from build123d import *

# Parameters (mm, degrees)
BOSS_EXTRUDE1_DEPTH                             = 5
CSK_FOR_M3_FLAT_HEAD_MACHINE_SCREW1_D           = 3.4
CSK_FOR_M3_FLAT_HEAD_MACHINE_SCREW1_DEPTH       = 10
CSK_FOR_M3_FLAT_HEAD_MACHINE_SCREW1_CSINK_D     = 4.2
CSK_FOR_M3_FLAT_HEAD_MACHINE_SCREW1_CSINK_ANGLE = 90
CSK_FOR_M3_FLAT_HEAD_MACHINE_SCREW1_TIP         = 1.021463052
CUT_EXTRUDE1_DEPTH                              = 2.762
SKETCH9_W                                       = 5
SKETCH9_H                                       = 5
CUT_EXTRUDE3_DEPTH                              = 1.5
SKETCH10_W                                      = 2
SKETCH10_H                                      = 2
CUT_EXTRUDE4_DEPTH                              = 3
CUT_EXTRUDE5_DEPTH                              = 3
CUT_EXTRUDE6_DEPTH                              = 3


with BuildPart() as part:
    # Sketch1 → Boss-Extrude1 (new body)
    with BuildSketch(Plane(origin=(0, 0, 0), x_dir=(0, 0, -1), z_dir=(1, 0, 0))):
        with BuildLine():
            Line((-36.25, 0.243748214), (36.25, 0.243748214))
            Line((36.25, 0.243748214), (36.25, 58.993748214))
            Line((36.25, 58.993748214), (39.75, 58.993748214))
            ThreePointArc((39.75, 58.993748214), (42.25, 61.493748214), (39.75, 63.993748214))
            Line((39.75, 63.993748214), (36.25, 63.993748214))
            Line((36.25, 63.993748214), (-10.25, 63.993748214))
            Line((-10.25, 63.993748214), (-36.25, 18.993748214))
            Line((-36.25, 18.993748214), (-36.25, 0.243748214))
        make_face()
        Polygon((31.25, 5.243748214), (-31.25, 5.243748214), (-31.25, 17.653143244), (-18.920674634, 38.992360224), (-7.364317129, 58.993748214), (31.25, 58.993748214), align=None, mode=Mode.SUBTRACT)
    extrude(amount=BOSS_EXTRUDE1_DEPTH)

    # CSK for M3 Flat Head Machine Screw1
    with Locations(Plane.ZY):
        with Locations((-39.75, 61.493748214)):
            CounterSinkHole(CSK_FOR_M3_FLAT_HEAD_MACHINE_SCREW1_D / 2, CSK_FOR_M3_FLAT_HEAD_MACHINE_SCREW1_CSINK_D / 2, depth=CSK_FOR_M3_FLAT_HEAD_MACHINE_SCREW1_DEPTH, counter_sink_angle=CSK_FOR_M3_FLAT_HEAD_MACHINE_SCREW1_CSINK_ANGLE)
            with Locations((0, 0, -(CSK_FOR_M3_FLAT_HEAD_MACHINE_SCREW1_DEPTH + CSK_FOR_M3_FLAT_HEAD_MACHINE_SCREW1_TIP / 2))):  # 118° drill point
                Cone(0, CSK_FOR_M3_FLAT_HEAD_MACHINE_SCREW1_D / 2, CSK_FOR_M3_FLAT_HEAD_MACHINE_SCREW1_TIP, mode=Mode.SUBTRACT)

    # Sketch6 → Cut-Extrude1 (cut)
    with BuildSketch(Plane(origin=(5, 0, 0), x_dir=(0, 0, -1), z_dir=(1, 0, 0))):
        Polygon((33.25, 60.993748214), (33.25, 3.243748214), (-33.25, 3.243748214), (-33.25, 18.189385232), (-8.518590277, 60.993748214), align=None)
    extrude(amount=-CUT_EXTRUDE1_DEPTH, mode=Mode.SUBTRACT)

    # Sketch9 → Cut-Extrude3 (cut)
    with BuildSketch(Plane.XY.offset(36.25)):
        with Locations((2.5, 2.743748214)):
            Rectangle(SKETCH9_W, SKETCH9_H)
    extrude(amount=-CUT_EXTRUDE3_DEPTH, mode=Mode.SUBTRACT)

    # Sketch10 → Cut-Extrude4 (cut)
    with BuildSketch(Plane(origin=(5, 0, 0), x_dir=(0, 0, -1), z_dir=(1, 0, 0))):
        with Locations((33.75, 61.993748214)):
            Rectangle(SKETCH10_W, SKETCH10_H)
    extrude(amount=-CUT_EXTRUDE4_DEPTH, mode=Mode.SUBTRACT)

    # Sketch13 → Cut-Extrude5 (cut)
    with BuildSketch(Plane(origin=(5, 0, 0), x_dir=(0, 0, -1), z_dir=(1, 0, 0))):
        Polygon((-8.75000025, 62.993748214), (-6.75, 62.993748214), (-6.750000265, 61.993748214), (-8.75000025, 61.993988423), align=None)
        Polygon((-11.135106519, 60.46294286), (-10.134551324, 62.194673006), (-9.26868625, 61.694395408), (-10.269241446, 59.962665262), align=None)
    extrude(amount=-CUT_EXTRUDE5_DEPTH, mode=Mode.SUBTRACT)

    # Sketch15 → Cut-Extrude6 (cut)
    with BuildSketch(Plane(origin=(5, 0, 0), x_dir=(0, 0, -1), z_dir=(1, 0, 0))):
        Polygon((-33.188472136, 22.293656216), (-33.938888532, 20.994858606), (-32.640090922, 20.244442209), (-31.889674526, 21.543239819), align=None)
    extrude(amount=-CUT_EXTRUDE6_DEPTH, mode=Mode.SUBTRACT)


solid = part.part
Could you check a few things on this model? Use its own coordinates, in mm. A direction names the side the tool comes from. Round coordinates to 2 decimals unless told otherwise and drop trailing zeros. Write each loop counter-clockwise with the first axis right and the second up, starting at its lowest first coordinate (ties: lowest second). Pieces come first, ordered by that corner, then holes. Notation, with made-up numbers: (-24.5, 58.25) - (14.5, 58.25) arc R34 ccw to (14.5, 91.25) - close; hole circle Ø3 at (86, 25.5). An arc over 180 degrees is marked (long way). Put each result on its own line as item: value. Start each with the question number.
(1) I want a section at C-C, the plane x = 4. Give the number of separate pieces and of enclosed holes in the cut face, plus the area to 3 significant figures.
(2) Will these pins go through, and if not, where does the flat tip stop? pin 1 (1 mm diameter, centred on y = 56, z = 15.5, fed in from +X); pin 2 (1.8 mm diameter, centred on x = 1.5, y = 25, fed in from +Z); pin 3 (2 mm diameter, centred on x = 4, y = 29, fed in from +Z); pin 4 (2 mm diameter, centred on x = 4, y = 62, fed in from +Z).
(3) For faces 1 (the flat face through (4, 62.994, -34)), 2 (the cylindrical face through (2.46, 61.44, -42.25)), 3 (the flat face through (2, 3, 34.75)), which set-ups out of +Z, -Z, +X, -X, +Y, -Y let a thin tool reach every point of the face, with its end or its side?
(4) I want a section at B-B, the plane y = 49. Please give me the cut outline in (x, z), plus the area to 3 significant figures.
(5) I need wall thicknesses on probe 1 along Y at (x, z) = (4.1, 7); probe 2 along Y at (x, z) = (2.55, -39.75); probe 3 along Y at (x, z) = (1.85, -17.5). Which ranges of each line are inside material? Lowest first, please.
(6) Thinking about a two-plate mould opening in Z: for faces 4 (the flat face through (2.465, 41.809, 23.068)), 5 (the flat face through (1, 11, 31.25)), 6 (the flat face through (5, 46, 18)), which applies, released by +Z, released by -Z, zero draft, split by the parting line, or undercut?
(7) I want a section at A-A, the plane z = -21.5. Please give me the cut outline in (x, y), plus the area to 3 significant figures.
Here are the results:
1. separate pieces: 1
1. enclosed holes: 5
1. area: 726 mm^2
2. pin 1: passes through
2. pin 2: stops at z = 33.3
2. pin 3: stops at z = 31.05
2. pin 4: stops at z = 11.98
3. face 1: +X
3. face 2: -Z, +X, -X
3. face 3: +Z, +X, -X, -Y
4. outline: (0, -36.25) - (5, -36.25) - (5, -33.25) - (2.24, -33.25) - (2.24, -31.25) - (0, -31.25) - close; (0, 13.14) - (2.24, 13.14) - (2.24, 15.45) - (5, 15.45) - (5, 18.91) - (0, 18.91) - close
4. area: 42.0 mm^2
5. probe 1: y = 0.24 to 3.24, 60.99 to 61.99, 62.99 to 63.99
5. probe 2: y = 58.99 to 59.79, 63.19 to 63.99
5. probe 3: y = 0.24 to 5.24, 58.99 to 63.99
6. face 4: released by +Z
6. face 5: undercut
6. face 6: zero draft
7. outline: (0, 0.24) - (5, 0.24) - (5, 3.24) - (2.24, 3.24) - (2.24, 5.24) - (0, 5.24) - close; (0, 58.99) - (2.24, 58.99) - (2.24, 60.99) - (5, 60.99) - (5, 63.99) - (0, 63.99) - close
7. area: 39.0 mm^2
